Work out the finished part from the listing and answer in its coordinate system (mm). A direction names the side the tool comes from. Give positions to 0.01 mm unless a question says otherwise; leave off trailing zeros. Write each loop counter-clockwise with the first axis right and the second up, starting at its lowest first coordinate (ties: lowest second). Pieces come first, ordered by that corner, then holes. Notation, with made-up numbers: (70.25, 55) - (88.25, 55) arc R28 cw to (88.25, 94) - close; hole circle Ø4 at (-15.5, -23.75). An arc over 180 degrees is marked (long way). Write item = value, one per line.
Autodesk Inventor part; units mm, degrees
ref_plane "YZ Plane" through (0, 0, 0) normal (1, 0, 0) x (0, 1, 0)
ref_plane "XZ Plane" through (0, 0, 0) normal (0, 1, 0) x (-1, 0, 0)
ref_plane "XY Plane" through (0, 0, 0) normal (0, 0, 1) x (1, 0, 0)
sketch "Sketch1" plane through (0, 0, 0) normal (0, 0, 1) x (1, 0, 0)
  line L0 (177.8, 0) -> (177.8, 152.4)
  line L1 (0, 152.4) -> (0, 0)
  line L2 (152.4, 152.4) -> (152.4, 155.575)
  line L3 (152.4, 155.575) -> (25.4, 155.575)
  line L4 (25.4, 155.575) -> (25.4, 152.4)
  line L5 (0, 152.4) -> (25.4, 152.4)
  line L6 (152.4, 152.4) -> (177.8, 152.4)
  line L7 (152.4, 0) -> (152.4, -3.175)
  line L8 (152.4, -3.175) -> (25.4, -3.175)
  line L9 (25.4, -3.175) -> (25.4, 0)
  line L10 (0, 0) -> (25.4, 0)
  line L11 (152.4, 0) -> (177.8, 0)
  dimension "d0" = 152.4
  dimension "d1" = 177.8
  dimension "d18" = 25.4
  dimension "d19" = 25.4
  dimension "d20" = 3.175
extrude "Extrusion3" add sketch "Sketch1" along normal blind 3.175
sketch "Sketch2" plane through (0, 0, 3.175) normal (0, 0, 1) x (1, 0, 0)
  line L0 (0, 152.4) -> (25.4, 152.4)
  line L1 (0, 0) -> (0, 152.4)
  line L2 (25.4, 0) -> (0, 0)
  line L3 (177.8, 0) -> (152.4, 0)
  line L4 (152.4, 152.4) -> (177.8, 152.4)
  line L5 (25.4, 152.4) -> (25.4, 155.575)
  line L6 (12.7, 152.4) -> (12.7, 139.7) construction
  line L7 (12.7, 139.7) -> (12.7, 114.3) construction
  line L8 (12.7, 114.3) -> (12.7, 88.9) construction
  line L9 (12.7, 88.9) -> (12.7, 63.5) construction
  line L10 (12.7, 63.5) -> (12.7, 38.1) construction
  line L11 (12.7, 38.1) -> (12.7, 12.7) construction
  line L12 (12.7, 12.7) -> (12.7, 0) construction
  circle A0 centre (12.7, 139.7) radius 2.3813
  circle A1 centre (12.7, 114.3) radius 2.3813
  circle A2 centre (12.7, 88.9) radius 2.3813
  circle A3 centre (12.7, 63.5) radius 2.3813
  circle A4 centre (12.7, 38.1) radius 2.3813
  circle A5 centre (12.7, 12.7) radius 2.3813
  line L13 (165.1, 152.4) -> (165.1, 139.7) construction
  line L14 (165.1, 139.7) -> (165.1, 114.3) construction
  line L15 (165.1, 114.3) -> (165.1, 88.9) construction
  line L16 (165.1, 88.9) -> (165.1, 63.5) construction
  line L17 (165.1, 63.5) -> (165.1, 38.1) construction
  line L18 (165.1, 38.1) -> (165.1, 12.7) construction
  line L19 (165.1, 12.7) -> (165.1, 0) construction
  circle A6 centre (165.1, 139.7) radius 2.3813
  circle A7 centre (165.1, 114.3) radius 2.3813
  circle A8 centre (165.1, 88.9) radius 2.3813
  circle A9 centre (165.1, 63.5) radius 2.3813
  circle A10 centre (165.1, 38.1) radius 2.3813
  circle A11 centre (165.1, 12.7) radius 2.3813
  dimension "d26" = 12.7
  dimension "d27" = 25.4
  dimension "d28" = 4.7625
  dimension "d29" = 12.7
  dimension "d30" = 25.4
  dimension "d31" = 4.7625
extrude "Extrusion4" cut sketch "Sketch2" against normal up to next
sketch "Sketch3" plane through (0, 0, 3.175) normal (0, 0, 1) x (1, 0, 0)
  line L0 (0, 0) -> (0, 152.4)
  line L1 (25.4, 0) -> (0, 0)
  circle A0 centre (76.2, 127) radius 3.175
  circle A1 centre (76.2, 12.7) radius 3.175
  dimension "d34" = 76.2
  dimension "d35" = 76.2
  dimension "d36" = 114.3
  dimension "d37" = 12.7
  dimension "d38" = 6.35
  dimension "d39" = 6.35
extrude "Extrusion5" cut sketch "Sketch3" against normal up to next
sketch "Sketch5" plane through (0, 0, 3.175) normal (0, 0, 1) x (1, 0, 0)
  line L0 (25.4, 155.575) -> (152.4, 155.575)
  line L1 (152.4, 155.575) -> (152.4, 152.4)
  line L2 (152.4, 152.4) -> (25.4, 152.4)
  line L3 (25.4, 152.4) -> (25.4, 155.575)
  line L4 (25.4, -3.175) -> (152.4, -3.175)
  line L5 (152.4, -3.175) -> (152.4, 0)
  line L6 (152.4, 0) -> (25.4, 0)
  line L7 (25.4, 0) -> (25.4, -3.175)
extrude "Extrusion7" add sketch "Sketch5" along normal blind 6.35
properties part number "DriveTrain_MotorMount" material "Aluminum-6061"
1. Find section A-A, the plane y = 63.5. Give the vertices of the cut face in (x, z) (3 decimals), then the cut area to 3 significant figures.
Solution:
outline = (0, 0) - (10.319, 0) - (10.319, 3.175) - (0, 3.175) - close; (15.081, 0) - (162.719, 0) - (162.719, 3.175) - (15.081, 3.175) - close; (167.481, 0) - (177.8, 0) - (177.8, 3.175) - (167.481, 3.175) - close
area = 534 mm^2
2. Straight lines are drawn through the part: line 1 (X direction, y = 139.7, z = 1.7); line 2 (Y direction, x = 126, z = 4.75) (3 decimals); line 3 (Z direction, x = 11, y = 125) (3 decimals). For each, find the intervals that lie inside material, in ascending order.
Solution:
line_1 = 0 to 10.32, 15.08 to 162.72, 167.48 to 177.8
line_2 = -3.175 to 0, 152.4 to 155.575
line_3 = 0 to 3.175
3. Given pin 1 (6 mm diameter, centred on x = 12.7, y = 63.5, fed in from +Z) (3 decimals); pin 2 (3.5 mm diameter, centred on x = 18, z = 1.5, fed in from +Y); pin 3 (2.5 mm diameter, centred on x = 160.5, z = 1, fed in from -Y), each flat-ended and moving along its own axis, determine where each tip first touches the part or whether it passes through.
Solution:
pin_1 = 3.175
pin_2 = 152.4
pin_3 = 0
4. Find section D-D, the plane y = 127. Give the vertices of the cut face in (x, z) (3 decimals), then the cut area to 3 significant figures.
Solution:
outline = (0, 0) - (73.025, 0) - (73.025, 3.175) - (0, 3.175) - close; (79.375, 0) - (177.8, 0) - (177.8, 3.175) - (79.375, 3.175) - close
area = 544 mm^2
5. For a pull along Y with two mould halves and no side action, classify faces 3 (the flat face through (90, -3.175, 5)), 4 (the flat face through (88, 77, 0)), 5 (the cylindrical face through (167.37, 13.42, 1.61)), 6 (the flat face through (90, 152.4, 6)) as pulls with the +Y half, pulls with the -Y half, needs draft (parallel to the pull), parting line crosses it, or undercut.
Solution:
face_3 = pulls with the -Y half
face_4 = needs draft
face_5 = undercut
face_6 = undercut
6. A tool of negligible diameter and unlimited length cuts with its end or side. For faces 1 (the cylindrical face through (167.3, 37.19, 1.61)), 2 (the flat face through (88, 77, 3.175)), from which of +Z, -Z, +X, -X, +Y, -Y can it reach the whole face along a straight path? Write none if from no direction.
Solution:
face_1 = +Z, -Z
face_2 = +Z, +X, -X
7. Find section C-C, the plane x = 12.7. Give the vertices of the cut face in (y, z) (3 decimals).
Solution:
outline = (0, 0) - (10.319, 0) - (10.319, 3.175) - (0, 3.175) - close; (15.081, 0) - (35.719, 0) - (35.719, 3.175) - (15.081, 3.175) - close; (40.481, 0) - (61.119, 0) - (61.119, 3.175) - (40.481, 3.175) - close; (65.881, 0) - (86.519, 0) - (86.519, 3.175) - (65.881, 3.175) - close; (91.281, 0) - (111.919, 0) - (111.919, 3.175) - (91.281, 3.175) - close; (116.681, 0) - (137.319, 0) - (137.319, 3.175) - (116.681, 3.175) - close; (142.081, 0) - (152.4, 0) - (152.4, 3.175) - (142.081, 3.175) - close
8. Find section B-B, the plane z = 5.75. Give the vertices of the cut face in (x, y) (3 decimals).
Solution:
outline = (25.4, -3.175) - (152.4, -3.175) - (152.4, 0) - (25.4, 0) - close; (25.4, 152.4) - (152.4, 152.4) - (152.4, 155.575) - (25.4, 155.575) - close
